```python
from build123d import *

# Parameters (mm, degrees)
F1_DEPTH = 3.175
F2_W     = 57.15
F2_H     = 101.6
F3_DEPTH = 6.351


with BuildPart() as f1:
    # F0 (on Front) → F1 (new body, symmetric)
    with BuildSketch(Plane.XZ):
        Polygon((98.933, 0), (-98.933, 0), (-244.983, -146.05), (244.983, -146.05), align=None)
    extrude(amount=F1_DEPTH, both=True)

    # F2 (on face) → F3 (cut, through all)
    with BuildSketch(Plane.XZ.offset(3.175)):
        with Locations((28.575, -95.25)):
            Rectangle(F2_W, F2_H)
        with Locations((-28.575, -95.25)):
            Rectangle(F2_W, F2_H)
    extrude(amount=-F3_DEPTH, mode=Mode.SUBTRACT)


solid = f1.part
```
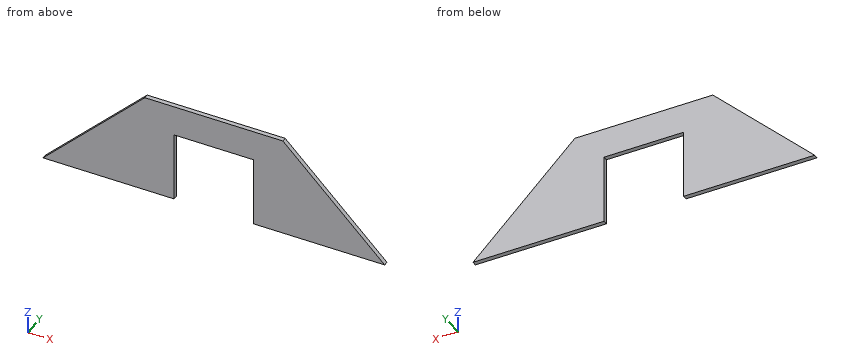
Design review of the part built by this model. Coordinates are the model's own, in mm. Coordinates: 2 decimals unless noted, no trailing zeros. Order: outer loops, then holes, each group sorted by start corner. A loop starts at its lowest first (then second) coordinate and runs counter-clockwise, first axis right, second up. Notation, with made-up numbers: (-34.75, 33) - (-11.75, 33) arc R15 cw to (-11.75, 55) - close; hole circle Ø2 at (82.5, 73). An arc over 180 degrees is marked (long way). One line per question, with ' | ' between items.
Q1. Consider section A-A, the plane z = -128. Give the boundary of the cut face in (x, y) (3 decimals).
Answer key:
outline: (-226.933, -3.175) - (-57.15, -3.175) - (-57.15, 3.175) - (-226.933, 3.175) - close; (57.15, -3.175) - (226.933, -3.175) - (226.933, 3.175) - (57.15, 3.175) - close
Q2. Consider section D-D, the plane z = -84. Give the boundary of the cut face in (x, y) (3 decimals), then the cut area to 3 significant figures.
Answer key:
outline: (-182.933, -3.175) - (-57.15, -3.175) - (-57.15, 3.175) - (-182.933, 3.175) - close; (57.15, -3.175) - (182.933, -3.175) - (182.933, 3.175) - (57.15, 3.175) - close | area: 1,600 mm2
Q3. Clearance check with a flat-ended pin moving along its axis: pin 1 Ø1.5 at (y, z) = (-0.5, -125.5) entering from -X. State where the tip first meets the part, or that it passes through.
Answer key:
pin 1: stops at x = -225.18
Q4. Consider section C-C, the plane x = -0.5. Give the boundary of the cut face in (y, z) (3 decimals), then the cut area to 3 significant figures.
Answer key:
outline: (-3.175, -44.45) - (3.175, -44.45) - (3.175, 0) - (-3.175, 0) - close | area: 282 mm2
Q5. To check wall thickness, follow line 1 along Z through (x, y) = (-41, 1.75); line 2 along X through (y, z) = (2.5, -117); line 3 along Z through (x, y) = (-156, -2). State the ranges of each line that lie inside material, in increasing order.
Answer key:
line 1: z = -44.45 to 0 | line 2: x = -215.93 to -57.15, 57.15 to 215.93 | line 3: z = -146.05 to -57.07
Q6. Consider section B-B, the plane y = -1.75. Give the boundary of the cut face in (x, z), then the cut area to 3 significant figures.
Answer key:
outline: (-244.98, -146.05) - (-57.15, -146.05) - (-57.15, -44.45) - (57.15, -44.45) - (57.15, -146.05) - (244.98, -146.05) - (98.93, 0) - (-98.93, 0) - close | area: 38,600 mm2
